Autodesk Inventor part; units mm, degrees
ref_plane "Work Plane1" through (-24.15, -24.15, 49.8) normal (0, 0, 1) x (1, 0, 0)
ref_plane "YZ Plane" through (0, 0, 0) normal (1, 0, 0) x (0, 1, 0)
ref_plane "XZ Plane" through (0, 0, 0) normal (0, 1, 0) x (-1, 0, 0)
sketch "Sketch1" plane through (0, 0, 0) normal (0, 0, 1) x (1, 0, 0)
  circle A0 centre (-21.9, -21.9) radius 1.875
  circle A1 centre (21.9, 21.9) radius 1.875
  circle A2 centre (21.9, -21.9) radius 1.875
  circle A3 centre (-21.9, 21.9) radius 1.875
  circle A4 centre (14.4, 20.8) radius 2.0675
  circle A5 centre (-14.4, -20.8) radius 2.0675
  circle A6 centre (14.4, -20.8) radius 2.0675
  circle A7 centre (20.8, -14.4) radius 2.0675
  line L0 (-17.05, 17.05) -> (-17.05, -17.05)
  line L1 (17.05, 17.05) -> (-17.05, 17.05)
  line L2 (17.05, -17.05) -> (17.05, 17.05)
  line L3 (-17.05, -17.05) -> (17.05, -17.05)
  circle A8 centre (20.8, 14.4) radius 2.0675
  circle A9 centre (-14.4, 20.8) radius 2.0675
  circle A10 centre (-20.8, -14.4) radius 2.0675
  circle A11 centre (-20.8, 14.4) radius 2.0675
  line L4 (-22.9, 24.15) -> (22.9, 24.15)
  arc A12 (-22.9, 24.15) -> (-24.15, 22.9) centre (-22.9, 22.9) ccw
  line L5 (-24.15, -22.9) -> (-24.15, 22.9)
  arc A13 (-24.15, -22.9) -> (-22.9, -24.15) centre (-22.9, -22.9) ccw
  line L6 (22.9, -24.15) -> (-22.9, -24.15)
  arc A14 (22.9, -24.15) -> (24.15, -22.9) centre (22.9, -22.9) ccw
  line L7 (24.15, 22.9) -> (24.15, -22.9)
  arc A15 (24.15, 22.9) -> (22.9, 24.15) centre (22.9, 22.9) ccw
  point P0 (0, 0)
ref_plane "Work Plane1" through (-24.15, -24.15, 49.8) normal (0, 0, 1) x (1, 0, 0)
extrude "Extrusion1" add sketch "Sketch1" along normal blind 1.5 from surface at 49.8 contours A0 | A1 | A2 | A3 | L1 L2 L3 L0 | L4 A15 L7 A14 L6 A13 L5 A12
sketch "Sketch2" plane through (-22.9, -24.15, 51.3) normal (0, 0, 1) x (1, 0, 0)
  arc A0 (-1.25, 1.25) -> (0, 0) centre (0, 1.25) ccw
  line L0 (45.8, 0) -> (0, 0)
  arc A1 (45.8, 0) -> (47.05, 1.25) centre (45.8, 1.25) ccw
  line L1 (47.05, 47.05) -> (47.05, 1.25)
  arc A2 (47.05, 47.05) -> (45.8, 48.3) centre (45.8, 47.05) ccw
  line L2 (0, 48.3) -> (45.8, 48.3)
  arc A3 (0, 48.3) -> (-1.25, 47.05) centre (0, 47.05) ccw
  line L3 (-1.25, 1.25) -> (-1.25, 47.05)
  circle A4 centre (2.1, 38.55) radius 2.0675
  circle A5 centre (2.1, 9.75) radius 2.0675
  circle A6 centre (8.5, 44.95) radius 2.0675
  circle A7 centre (43.7, 38.55) radius 2.0675
  circle A8 centre (43.7, 9.75) radius 2.0675
  circle A9 centre (37.3, 3.35) radius 2.0675
  circle A10 centre (8.5, 3.35) radius 2.0675
  circle A11 centre (37.3, 44.95) radius 2.0675
  arc A12 (47.9, 47.05) -> (45.8, 49.15) centre (45.8, 47.05) ccw
  line L4 (47.9, 47.05) -> (47.9, 1.25)
  arc A13 (45.8, -0.85) -> (47.9, 1.25) centre (45.8, 1.25) ccw
  line L5 (45.8, -0.85) -> (0, -0.85)
  arc A14 (-2.1, 1.25) -> (0, -0.85) centre (0, 1.25) ccw
  line L6 (-2.1, 1.25) -> (-2.1, 47.05)
  arc A15 (0, 49.15) -> (-2.1, 47.05) centre (0, 47.05) ccw
  line L7 (0, 49.15) -> (45.8, 49.15)
  line L8 (47.05, 1.25) -> (45.8, 1.25)
  line L9 (45.8, 1.25) -> (45.8, -0.85)
  line L10 (45.8, -0.85) -> (47.05, -0.85)
  line L11 (47.05, -0.85) -> (47.05, 1.25)
  line L12 (-1.25, 1.25) -> (0, 1.25)
  line L13 (0, 1.25) -> (0, -0.85)
  line L14 (0, -0.85) -> (-1.25, -0.85)
  line L15 (-1.25, -0.85) -> (-1.25, 1.25)
  line L16 (-1.25, 47.05) -> (0, 47.05)
  line L17 (0, 47.05) -> (0, 49.15)
  line L18 (0, 49.15) -> (-1.25, 49.15)
  line L19 (-1.25, 49.15) -> (-1.25, 47.05)
  line L20 (47.05, 47.05) -> (45.8, 47.05)
  line L21 (45.8, 47.05) -> (45.8, 49.15)
  line L22 (45.8, 49.15) -> (47.05, 49.15)
  line L23 (47.05, 49.15) -> (47.05, 47.05)
  point P0 (22.9, 24.15)
  dimension "d2" = 0.85
extrude "Extrusion2" add sketch "Sketch2" against normal blind 1.5 contours A0 L13 A14 L15 | L0 L9 L5 L13 | L19 A15 L17 A3 | A14 L14 L15 | A1 L11 A13 L9 | L17 L7 L21 L2 | L19 L18 A15 | A13 L11 L10 | L21 A12 L23 A2 | L22 L23 A12
pattern_linear "Rectangular Pattern1" count 4 spacing 50 along (0, 1, 0) of "Extrusion1", "Extrusion2"
chamfer "Chamfer1" distance 1.5 angle 45 2 edges at (0, -25, 51.3) (0, 175, 51.3)
properties part number "Panel Top 1x4"
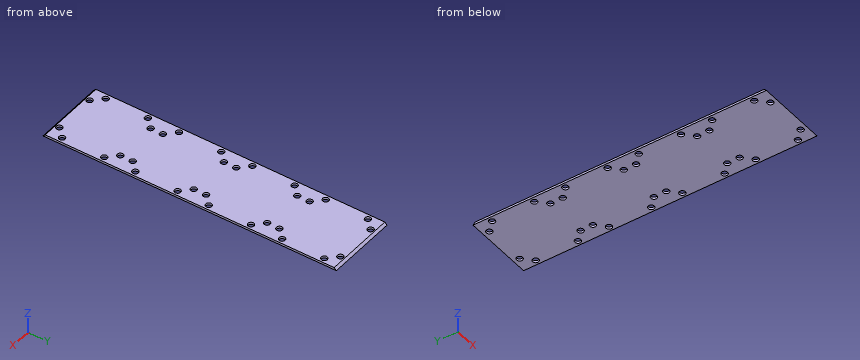
CAD build for the part. Positions are in the model's coordinates, mm. Round coordinates to 2 decimals unless told otherwise and drop trailing zeros. Write each loop counter-clockwise with the first axis right and the second up, starting at its lowest first coordinate (ties: lowest second). Pieces come first, ordered by that corner, then holes. Notation, with made-up numbers: (-9.75, 60.5) -> (46.25, 60.5) arc R9 ccw to (46.25, 75.5) -> close; hole circle Ø8 at (66, -14). An arc over 180 degrees is marked (long way). Answer in a Markdown table with one row per item. Add a question column.
Item 1: Drill centre lines: line 1 (X direction, y = 120.5, z = 50.3); line 2 (X direction, y = 164.4, z = 50.3); line 3 (Y direction, x = 8, z = 50.5). Where is each one in solid material? Low to high. Write a range as from..to.
Item 2: Saw through at B-B, the plane x = 20.8. Count the separate pieces of the cut face and the enclosed holes in it, then the cut area to 3 significant figures.
Item 3: Saw through at A-A, the plane y = 129.2. Write the cut outline in (x, z).
Findings below:
| question | item | result |
|---|---|---|
| 1 | line 1 | x = -24.15..-16.45, -12.35..12.35, 16.45..24.15 |
| 1 | line 2 | x = -24.15..-22.87, -18.73..18.73, 22.87..24.15 |
| 1 | line 3 | y = -24.3..174.3 |
| 2 | separate pieces | 9 |
| 2 | enclosed holes | 0 |
| 2 | area | 248 mm^2 |
| 3 | outline | (-24.15, 49.8) -> (-16.47, 49.8) -> (-16.47, 51.3) -> (-24.15, 51.3) -> close; (-12.33, 49.8) -> (12.33, 49.8) -> (12.33, 51.3) -> (-12.33, 51.3) -> close; (16.47, 49.8) -> (24.15, 49.8) -> (24.15, 51.3) -> (16.47, 51.3) -> close |
